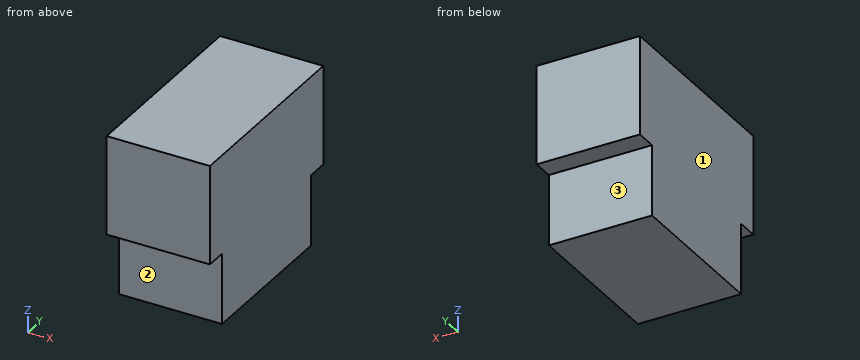
```python
from build123d import *

# Parameters (mm, degrees)
F0_W     = 7.3
F0_H     = 14
F1_DEPTH = 12
F2_W     = 1.5
F2_H     = 5
F3_DEPTH = 25


with BuildPart() as f1:
    # F0 (on Top) → F1 (new body)
    with BuildSketch(Plane.XY):
        Rectangle(F0_W, F0_H)
    extrude(amount=F1_DEPTH)

    # F2 (on face) → F3 (cut)
    with BuildSketch(Plane.YZ.offset(3.65)):
        with Locations((-6.25, 2.5)):
            Rectangle(F2_W, F2_H)
        with Locations((6.25, 2.5)):
            Rectangle(F2_W, F2_H)
    extrude(amount=-F3_DEPTH, mode=Mode.SUBTRACT)


solid = f1.part
```
Input: part model. Units: mm. Frame: model coordinates. Face numbers are marked on the shaded views. A direction names the side the tool comes from. Give positions to 0.01 mm unless a question says otherwise; leave off trailing zeros. Loops run counter-clockwise (first coordinate to the right, second up) from the corner with the lowest first, then second, coordinate; pieces in that order, holes last.
1) Section query A-A on x = -2.5. Return the cut outline in (y, z), and give its area (3 significant figures).
A:
outline: (-7, 5) - (-5.5, 5) - (-5.5, 0) - (5.5, 0) - (5.5, 5) - (7, 5) - (7, 12) - (-7, 12) - close
area: 153 mm2
2) Reachability of the marked faces 1, 2 and 3 from +Z, -Z, +X, -X, +Y, -Y: full face, straight path, thin tool, end or side. Return the list, or none.
A:
face 1: +Z, -Z, -X, +Y, -Y
face 2: -Z, +X, -X, -Y
face 3: -Z, +X, -X, +Y
3) Line query: L1, parallel to Z at x = 0, y = 6.25; L2, parallel to Y at x = 2.25, z = 3.75. Output: solid intervals per line, ascending.
A:
L1: z = 5 to 12
L2: y = -5.5 to 5.5
4) Section query B-B on z = 3. Return the cut outline in (x, y).
A:
outline: (-3.65, -5.5) - (3.65, -5.5) - (3.65, 5.5) - (-3.65, 5.5) - close
5) Contact query for flat-ended pins moving along their axis: pin 1 (3 mm diameter, centred on x = 0, z = 1.5, fed in from -Y); pin 2 (0.8 mm diameter, centred on x = -0.5, y = -6, fed in from -Z); pin 3 (1.5 mm diameter, centred on x = 0, z = 3.5, fed in from +Y). Output: stop coordinate, or through.
A:
pin 1: stops at y = -5.5
pin 2: stops at z = 5
pin 3: stops at y = 5.5
